```python
from build123d import *

# Parameters (mm, degrees)
BOSS_EXTRUDE1_DEPTH       = 13.6
BOSS_EXTRUDE2_DEPTH       = 13.6
CHAMFER1_SIZE             = 50
CHAMFER1_SIZE2            = 2.620388964
F_3_0MM_DOWEL_HOLE1_D     = 3.2
F_3_0MM_DOWEL_HOLE1_DEPTH = 1.2
F_3_0MM_DOWEL_HOLE2_D     = 3.2
F_3_0MM_DOWEL_HOLE2_DEPTH = 1.2
F_3_0MM_DOWEL_HOLE3_D     = 3.2
F_3_0MM_DOWEL_HOLE3_DEPTH = 1.2


with BuildPart() as part:
    # wrist → Boss-Extrude1 (new body)
    with BuildSketch(Plane(origin=(0, 0, 0), x_dir=(1, 0, 0), z_dir=(0, 1, 0))):
        Polygon((165.988080985, -4.817824349), (165.988080985, 22.235679058), (143.430369308, 20.475150048), (134.081949487, 5.381860359), (111.510829699, 5.381860359), (93.059430407, 10.480109343), (76.207852469, 10.480109343), (37.653795388, -4.817824349), align=None)
    extrude(amount=BOSS_EXTRUDE1_DEPTH)

    # wrist<5> → Boss-Extrude2 (add)
    with BuildSketch(Plane(origin=(0, 0, 0), x_dir=(1, 0, 0), z_dir=(0, 1, 0))):
        Polygon((165.988080985, -60.618139641), (165.988080985, -4.817824349), (37.653795388, -4.817824349), (75.231684079, -60.618139641), align=None)
    extrude(amount=BOSS_EXTRUDE2_DEPTH)

    # Chamfer1
    chamfer1_edges = [part.edges().sort_by_distance(p)[0] for p in [
        (120.609882532, 13.6, 60.618139641),
    ]]
    chamfer1_side = [part.faces().sort_by_distance(p)[0] for p in [
        (112.052751193, 13.6, 23.244648168),
    ]]
    chamfer(chamfer1_edges, length=CHAMFER1_SIZE, length2=CHAMFER1_SIZE2, reference=chamfer1_side[0])

    # Fillet1
    # an asymmetric fillet: 11, 3 mm, written as the material it takes off along each edge
    with BuildSketch(Plane(origin=(48.087002909, 10.979611036, 60.618139641), x_dir=(0, 0.05233595624294356, -0.9986295347545739), z_dir=(1, 0, 0))) as fillet1_piece_1:
        with BuildLine():
            Bezier((2.427631466, 0), (0, 0), (-0.568257138, -10.842992131), weights=[1, 0.725374371, 1])
            Line((-0.568257138, -10.842992131), (0, 0))
            Line((0, 0), (2.427631466, 0))
        make_face()
    extrude(amount=145.045759247, mode=Mode.SUBTRACT)

    # Ø3.0mm Dowel Hole1
    with Locations(Plane(origin=(-0.719959147, 0, -9.224858415), x_dir=(-0.9969682889311796, 0, 0.07780893821172487), z_dir=(-0.07780893821172487, 0, -0.9969682889311796))):
        with Locations((-155.901833608, 6.8)):
            Hole(F_3_0MM_DOWEL_HOLE1_D / 2, depth=F_3_0MM_DOWEL_HOLE1_DEPTH)

    # Ø3.0mm Dowel Hole2
    with Locations(Plane(origin=(0, 0, -5.381860359), x_dir=(-1, 0, 0), z_dir=(0, 0, -1))):
        with Locations((-122.796389593, 6.8)):
            Hole(F_3_0MM_DOWEL_HOLE2_D / 2, depth=F_3_0MM_DOWEL_HOLE2_DEPTH)

    # Ø3.0mm Dowel Hole3
    with Locations(Plane(origin=(0, 0, -10.480109343), x_dir=(-1, 0, 0), z_dir=(0, 0, -1))):
        with Locations((-84.633641438, 6.8)):
            Hole(F_3_0MM_DOWEL_HOLE3_D / 2, depth=F_3_0MM_DOWEL_HOLE3_DEPTH)


solid = part.part
```
Build history of the part. All positions in model axes, mm. A direction names the side the tool comes from. Coordinates: 2 decimals unless noted, no trailing zeros. Write each loop counter-clockwise with the first axis right and the second up, starting at its lowest first coordinate (ties: lowest second). Pieces come first, ordered by that corner, then holes.
1. Band-saw the part on A-A, the plane z = 49. Give the cut face in (x, y), and give its area (3 significant figures).
Answer block:
outline: (67.41, 0) - (165.99, 0) - (165.99, 11.59) - (67.41, 11.59) - close
area: 1,140 mm2
2. Pull direction Y, two halves, no side cores. Call faces 4 (the cylindrical face through (124.274, 6.187, -4.773)), 5 (the flat face through (85, 5, -10.48)), 6 (the flat face through (116.728, 12.336, 34.739)): released by +Y, released by -Y, zero draft, split by the parting line, or undercut.
Answer block:
face 4: undercut
face 5: zero draft
face 6: released by +Y
3. Drill centre lines: probe 1 along X at (y, z) = (6.5, 25); probe 2 along Z at (x, y) = (136, 1.5); probe 3 along Z at (x, y) = (59.5, 2). Where is each one in solid material? Low to high.
Answer block:
probe 1: x = 51.25 to 165.99
probe 2: z = -8.48 to 60.6
probe 3: z = -3.85 to 37.26
4. Drop flat-ended pins along their axis: pin 1 (8 mm diameter, centred on x = 131, z = -11.5, fed in from +Y); pin 2 (5 mm diameter, centred on x = 122.8, y = 6.8, fed in from -Z); pin 3 (3.5 mm diameter, centred on x = 84.5, y = 7.5, fed in from -Z); pin 4 (4 mm diameter, centred on y = 9, z = 13, fed in from -X). Give the stop position or say it passes through.
Answer block:
pin 1: passes through
pin 2: stops at z = -5.38
pin 3: stops at z = -10.48
pin 4: stops at x = 41.82
5. 3-axis set-ups, long thin cutter, end or side, ignore diameter. For faces 1 (the flat face through (85, 7, -9.28)), 2 (the flat face through (115, 0, 19)), 3 (the flat face through (138.8, 6.7, -13)): which of +Z, -Z, +X, -X, +Y, -Y reach the whole face in a straight line?
Answer block:
face 1: -Z
face 2: +Z, -Z, +X, -X, -Y
face 3: -Z, +Y, -Y
6. Band-saw the part on B-B, the plane z = 33.5. Give the cut face in (x, y).
Answer block:
outline: (56.97, 0) - (165.99, 0) - (165.99, 12.4) - (56.97, 12.4) - close
